For this review, take the finished solid that the model builds, in its own axes (mm). A direction names the side the tool comes from. Round coordinates to 2 decimals unless told otherwise and drop trailing zeros. Write each loop counter-clockwise with the first axis right and the second up, starting at its lowest first coordinate (ties: lowest second). Pieces come first, ordered by that corner, then holes. Notation, with made-up numbers: M 5.25,77 L 18.25,77 A13 ccw 18.25,88 Z; hole C 11.5,22 d7. An arc over 180 degrees is marked long. Answer in a Markdown table with one row per item.
```python
from build123d import *

# Parameters (mm, degrees)
PAD011_DEPTH    = 4.5
PAD025_DEPTH    = 100.98
SKETCH030_R     = 3.8
PAD026_DEPTH    = 37.4
SKETCH031_W     = 3.5
SKETCH031_H     = 10.5
PAD027_DEPTH    = 10
CHAMFER009_SIZE = 3.49
SKETCH043_R     = 8
POCKET003_DEPTH = 5
PAD029_DEPTH    = 4.5
SKETCH032_W     = 70
SKETCH032_H     = 24.7
PAD028_DEPTH    = 10
SKETCH041_W     = 10
SKETCH041_H     = 10
PAD037_DEPTH    = 100.5
PAD039_DEPTH    = 5.25
FILLET001_R     = 2
CHAMFER015_SIZE = 1
PAD038_DEPTH    = 5.25
FILLET_R        = 2
CHAMFER014_SIZE = 1
PAD010_DEPTH    = 70
CHAMFER011_SIZE = 2.125
CHAMFER013_SIZE = 2.125
SKETCH045_R     = 5.5
SKETCH045_W     = 7
SKETCH045_H     = 12
POCKET005_DEPTH = 5
SKETCH046_W     = 11
SKETCH046_H     = 3
POCKET006_DEPTH = 5
POCKET007_DEPTH = 5


with BuildPart() as band:
    # Sketch013 → Pad011 (new body)
    with BuildSketch(Plane.XY.offset(27.45)):
        Polygon((-35, 0), (-35, -24.7), (35, -24.7), (35, 0), (34, 0), (34, -23.7), (20, -23.7), (20, -22.7), (-20, -22.7), (-20, -23.7), (-34, -23.7), (-34, 0), align=None)
    extrude(amount=PAD011_DEPTH)


with BuildPart() as boardcover:
    # Sketch029 → Pad025 (new body)
    with BuildSketch(Plane.XY.offset(34.7)):
        Polygon((-35, 0), (-35, -24.7), (35, -24.7), (35, 0), (31.5, 0), (31.5, -21.2), (-31.5, -21.2), (-31.5, 0), align=None)
    extrude(amount=PAD025_DEPTH)

    # Sketch030 (on Face6 of Pad025) → Pad026 (join)
    with BuildSketch(Plane(origin=(0, -21.2, 0), x_dir=(-1, 0, 0), z_dir=(0, 1, 0))):
        with Locations((-22.225, 129.005)):
            Circle(SKETCH030_R)
        with Locations((22.225, 129.005)):
            Circle(SKETCH030_R)
        with Locations((-22.225, 41.375)):
            Circle(SKETCH030_R)
        with Locations((22.225, 41.375)):
            Circle(SKETCH030_R)
    extrude(amount=PAD026_DEPTH)

    # Sketch031 → Pad027 (join)
    with BuildSketch(Plane.XZ.offset(-5)):
        with Locations((29.75, 130.43)):
            Rectangle(SKETCH031_W, SKETCH031_H)
        with Locations((-29.75, 130.43)):
            Rectangle(SKETCH031_W, SKETCH031_H)
        with Locations((29.75, 39.95)):
            Rectangle(SKETCH031_W, SKETCH031_H)
        with Locations((-29.75, 39.95)):
            Rectangle(SKETCH031_W, SKETCH031_H)
    extrude(amount=PAD027_DEPTH)

    # Chamfer009
    chamfer009_edges = [boardcover.edges().sort_by_distance(p)[0] for p in [
        (28, -5, 130.43),
        (28, -5, 39.95),
        (-28, -5, 130.43),
        (-28, -5, 39.95),
    ]]
    chamfer(chamfer009_edges, length=CHAMFER009_SIZE)

    # Sketch043 (on Face3 of Boolean005) → Pocket003 (cut)
    with BuildSketch(Plane(origin=(0, -24.7, 10), x_dir=(1, 0, 0), z_dir=(0, -1, 0))):
        with Locations((0, 55)):
            Circle(SKETCH043_R)
        with BuildLine():
            Line((3.641143, 64.313543), (18.302914, 86.985827))
            Line((18.302914, 86.985827), (21.661771, 84.813713))
            Line((21.661771, 84.813713), (7, 62.141428))
            ThreePointArc((7, 62.141428), (5.430286, 63.397142), (3.641143, 64.313543))
        make_face()
        with BuildLine():
            ThreePointArc((15.712042, 88.498235), (3.658274, 91.818705), (-8.813211, 90.935043))
            Line((-9.765986, 94.819914), (-8.813211, 90.935043))
            Line((-21.351919, 86.31544), (-9.765986, 94.819914))
            Line((-7.145856, 84.136519), (-21.351919, 86.31544))
            Line((-8.098631, 88.02139), (-7.145856, 84.136519))
            ThreePointArc((14.438081, 85.782167), (3.361649, 88.833405), (-8.098631, 88.02139))
            Line((15.712042, 88.498235), (14.438081, 85.782167))
        make_face()
    extrude(amount=-POCKET003_DEPTH, mode=Mode.SUBTRACT)


with BuildPart() as body015:
    # Sketch033 → Pad029 (new body)
    with BuildSketch(Plane.XY.offset(138.43)):
        Polygon((-35, 0), (-35, -24.7), (35, -24.7), (35, 0), (34, 0), (34, -23.7), (-34, -23.7), (-34, 0), align=None)
    extrude(amount=PAD029_DEPTH)


with BuildPart() as zip2:
    # Sketch032 → Pad028 (new body)
    with BuildSketch(Plane.XY.offset(135.68)):
        with Locations((0, -12.35)):
            Rectangle(SKETCH032_W, SKETCH032_H)
    extrude(amount=PAD028_DEPTH)

    # Boolean006: cut Body015
    add(body015.part, mode=Mode.SUBTRACT)

    # Sketch041 (on Face8 of Boolean006) → Pad037 (join)
    with BuildSketch(Plane.XY.offset(145.68)):
        with Locations((-26.5, -17.25)):
            Rectangle(SKETCH041_W, SKETCH041_H)
        with Locations((26.5, -17.25)):
            Rectangle(SKETCH041_W, SKETCH041_H)
    extrude(amount=PAD037_DEPTH)


with BuildPart() as body021:
    # Sketch050 → Pad039 (new body)
    with BuildSketch(Plane(origin=(0, -17.5, 0), x_dir=(-1, 0, 0), z_dir=(0, 1, 0))):
        Polygon((35, 70.5), (51, 70.5), (51, 201.1), (35, 201.1), (31.5, 201.1), (31.5, 211.6), (35, 211.6), (51, 211.6), (51, 222.1), (61.5, 222.1), (61.5, 49.5), (51, 49.5), (51, 60), (35, 60), align=None)
    extrude(amount=PAD039_DEPTH)

    # Fillet001
    fillet001_edges = [body021.edges().sort_by_distance(p)[0] for p in [
        (-43, -17.5, 211.6),
        (-33.25, -17.5, 211.6),
        (-43, -12.25, 211.6),
        (-33.25, -12.25, 211.6),
        (-43, -12.25, 60),
        (-43, -17.5, 60),
    ]]
    fillet(fillet001_edges, radius=FILLET001_R)

    # Chamfer015
    chamfer015_edges = [body021.edges().sort_by_distance(p)[0] for p in [
        (-51, -14.875, 222.1),
        (-56.25, -17.5, 222.1),
        (-56.25, -12.25, 222.1),
        (-61.5, -14.875, 222.1),
        (-61.5, -17.5, 135.8),
        (-61.5, -12.25, 135.8),
        (-51, -14.875, 49.5),
        (-56.25, -17.5, 49.5),
        (-56.25, -12.25, 49.5),
        (-61.5, -14.875, 49.5),
    ]]
    chamfer(chamfer015_edges, length=CHAMFER015_SIZE)


with BuildPart() as body020:
    # Sketch049 → Pad038 (new body)
    with BuildSketch(Plane.XZ.offset(12.25)):
        Polygon((35, 70.5), (51, 70.5), (51, 201.1), (35, 201.1), (31.5, 201.1), (31.5, 211.6), (35, 211.6), (51, 211.6), (51, 222.1), (61.5, 222.1), (61.5, 49.5), (51, 49.5), (51, 60), (35, 60), align=None)
    extrude(amount=PAD038_DEPTH)

    # Fillet
    fillet_edges = [body020.edges().sort_by_distance(p)[0] for p in [
        (43, -17.5, 60),
        (43, -12.25, 60),
        (33.25, -17.5, 211.6),
        (33.25, -12.25, 211.6),
        (43, -12.25, 211.6),
        (43, -17.5, 211.6),
    ]]
    fillet(fillet_edges, radius=FILLET_R)

    # Chamfer014
    chamfer014_edges = [body020.edges().sort_by_distance(p)[0] for p in [
        (51, -14.875, 222.1),
        (56.25, -12.25, 222.1),
        (56.25, -17.5, 222.1),
        (61.5, -17.5, 135.8),
        (61.5, -14.875, 222.1),
        (61.5, -12.25, 135.8),
        (61.5, -14.875, 49.5),
        (56.25, -12.25, 49.5),
        (56.25, -17.5, 49.5),
        (51, -14.875, 49.5),
    ]]
    chamfer(chamfer014_edges, length=CHAMFER014_SIZE)


with BuildPart() as plate:
    # Sketch012 → Pad010 (new body)
    with BuildSketch(Plane.YZ.offset(-35)):
        Polygon((-24.7, 20.45), (-20.45, 24.7), (0, 24.7), (0, 34.7), (-24.7, 34.7), align=None)
    extrude(amount=PAD010_DEPTH)

    # Boolean002: cut Band
    add(band.part, mode=Mode.SUBTRACT)

    # Boolean009: union BoardCover, Zip2
    add(boardcover.part)
    add(zip2.part)

    # Chamfer011
    chamfer011_edges = [plate.edges().sort_by_distance(p)[0] for p in [
        (-35, -24.7, 23.95),
        (-34, -23.7, 29.7),
        (-35, -24.7, 33.325),
        (-35, -24.7, 85.19),
        (-34, -23.7, 140.68),
        (-35, -24.7, 137.055),
        (-35, -24.7, 144.305),
        (35, -24.7, 144.305),
        (34, -23.7, 140.68),
        (35, -24.7, 137.055),
        (35, -24.7, 85.19),
        (35, -24.7, 33.325),
        (34, -23.7, 29.7),
        (35, -24.7, 23.95),
    ]]
    chamfer(chamfer011_edges, length=CHAMFER011_SIZE)

    # Chamfer013
    chamfer013_edges = [plate.edges().sort_by_distance(p)[0] for p in [
        (-31.5, -22.25, 195.93),
        (-21.5, -22.25, 195.93),
        (21.5, -22.25, 195.93),
        (31.5, -22.25, 195.93),
    ]]
    chamfer(chamfer013_edges, length=CHAMFER013_SIZE)

    # Sketch045 (on Face54 of Chamfer012) → Pocket005 (cut)
    with BuildSketch(Plane(origin=(-35, 0, 0), x_dir=(0, -1, 0), z_dir=(-1, 0, 0))):
        with Locations((-9.7, 101.7)):
            Circle(SKETCH045_R)
        with Locations((-2.34, 81.38)):
            Rectangle(SKETCH045_W, SKETCH045_H)
    extrude(amount=-POCKET005_DEPTH, mode=Mode.SUBTRACT)

    # Sketch046 (on Face97 of Pocket005) → Pocket006 (cut)
    with BuildSketch(Plane.XZ.offset(24.7)):
        with Locations((-12.7, 44)):
            Rectangle(SKETCH046_W, SKETCH046_H)
        with Locations((12.7, 44)):
            Rectangle(SKETCH046_W, SKETCH046_H)
    extrude(amount=-POCKET006_DEPTH, mode=Mode.SUBTRACT)

    # Sketch048 → Pocket007 (cut)
    with BuildSketch(Plane.YZ.offset(-24.5)):
        Polygon((-24.7, 138.43), (-24.7, 131.43), (-22.7, 138.43), (-22.7, 142.93), (-24.7, 142.93), align=None)
        Polygon((-22.7, 27.45), (-24.7, 20.45), (-24.7, 27.45), (-24.7, 31.95), (-22.7, 31.95), align=None)
    extrude(amount=-POCKET007_DEPTH, mode=Mode.SUBTRACT)

    # Boolean011: union Body021, Body020
    add(body021.part)
    add(body020.part)


solid = plate.part
```
Q1. Machinability: for faces 1 (the face through (-28, 2, 40)), 2 (the face through (35, -11, 26)), 3 (the face through (52, -12.25, 155)), 4 (the face through (14.434, -22.974, 83.636)), which of the approach directions +Z, -Z, +X, -X, +Y, -Y give a long, thin tool a straight path to every point of the face, cutting with its end or side? Answer none if there is none.
Found:
| item | result |
|---|---|
| face 1 | +Y |
| face 2 | -Z, +X, +Y, -Y |
| face 3 | +Z, +X, +Y |
| face 4 | +Y, -Y |
Q2. Insertion check: P1, Ø1, axis at x = -20, z = 154, coming from the -Y side; P2, Ø2, axis at x = 24, z = 30.5, coming from the -Y side; P3, Ø1.8, axis at x = 29.5, y = 1.5, coming from the -Z side; P4, Ø10.5, axis at x = 3, y = -11.5, coming from the -Z side. Each pin has a flat end and moves straight along its axis. Give the tip position at first contact, or say it passes through.
Found:
| item | result |
|---|---|
| P1 | through |
| P2 | y = -23.7 |
| P3 | z = 34.7 |
| P4 | z = 24.7 |
Q3. Take a section at B-B (x = -48). State the section outline as (y, z) points, then the cut area to 3 significant figures.
Found:
| item | result |
|---|---|
| outline | M -17.5,62 A2 ccw -15.5,60 L -14.25,60 A2 ccw -12.25,62 L -12.25,70.5 L -17.5,70.5 Z; M -17.5,201.1 L -12.25,201.1 L -12.25,209.6 A2 ccw -14.25,211.6 L -15.5,211.6 A2 ccw -17.5,209.6 Z |
| area | 107 mm² |
Q4. Mouldability with a two-part tool opening along Z and no side actions: class faces 5 (the face through (-22, 16.2, 41)), 6 (the face through (-3, -24, 142.93)) as +Z half, -Z half, draft (parallel to the pull), parting line (faces both ways), or undercut.
Found:
| item | result |
|---|---|
| face 5 | draft |
| face 6 | undercut |
Q5. For probe 1 along X at (y, z) = (-15.5, 152); probe 2 along Z at (x, y) = (0, -23.45); probe 3 along X at (y, z) = (-4.5, 109), list the stretches that pass through material, from the lowest coordinate up.
Found:
| item | result |
|---|---|
| probe 1 | -61.5 to -51, -31.5 to -21.5, 21.5 to 31.5, 51 to 61.5 |
| probe 2 | 21.7 to 27.45, 31.95 to 57, 73 to 99, 102 to 145.68 |
| probe 3 | -35 to -31.5, 31.5 to 35 |
Q6. Take a section at D-D (x = 0). State the section outline as (y, z) points.
Found:
| item | result |
|---|---|
| outline | M -24.7,20.45 L -20.45,24.7 L 0,24.7 L 0,34.7 L -21.2,34.7 L -21.2,57 L -24.7,57 L -24.7,31.95 L -22.7,31.95 L -22.7,27.45 L -24.7,27.45 Z; M -24.7,73 L -21.2,73 L -21.2,99 L -24.7,99 Z; M -24.7,102 L -21.2,102 L -21.2,135.68 L 0,135.68 L 0,145.68 L -24.7,145.68 L -24.7,142.93 L -23.7,142.93 L -23.7,138.43 L -24.7,138.43 Z |
Q7. Take a section at C-C (z = 153.5). State the section outline as (x, y) points (3 decimals).
Found:
| item | result |
|---|---|
| outline | M -61.5,-16.5 L -60.5,-17.5 L -51,-17.5 L -51,-12.25 L -60.5,-12.25 L -61.5,-13.25 Z; M -31.5,-20.125 L -29.375,-22.25 L -23.625,-22.25 L -21.5,-20.125 L -21.5,-12.25 L -31.5,-12.25 Z; M 21.5,-20.125 L 23.625,-22.25 L 29.375,-22.25 L 31.5,-20.125 L 31.5,-12.25 L 21.5,-12.25 Z; M 51,-17.5 L 60.5,-17.5 L 61.5,-16.5 L 61.5,-13.25 L 60.5,-12.25 L 51,-12.25 Z |
Q8. Take a section at A-A (z = 65). State the section outline as (x, y) points (3 decimals).
Found:
| item | result |
|---|---|
| outline | M -61.5,-16.5 L -60.5,-17.5 L -35,-17.5 L -35,-22.575 L -32.875,-24.7 L -8,-24.7 L -8,-21.2 L -31.5,-21.2 L -31.5,0 L -35,0 L -35,-12.25 L -60.5,-12.25 L -61.5,-13.25 Z; M 8,-24.7 L 32.875,-24.7 L 35,-22.575 L 35,-17.5 L 60.5,-17.5 L 61.5,-16.5 L 61.5,-13.25 L 60.5,-12.25 L 35,-12.25 L 35,0 L 31.5,0 L 31.5,-21.2 L 8,-21.2 Z |
